Check sheet for the modelled part. Datum: model origin and axes. Units: mm. A direction names the side the tool comes from. Round coordinates to 2 decimals unless told otherwise and drop trailing zeros. Loops run counter-clockwise (first coordinate to the right, second up) from the corner with the lowest first, then second, coordinate; pieces in that order, holes last. Notation, with made-up numbers: (52.5, 72) - (81.5, 72) arc R6 ccw to (81.5, 81) - close; hole circle Ø4 at (-6, 0). An arc over 180 degrees is marked (long way). Return JSON: item names as keys, results as strings.
Autodesk Inventor part; units mm, degrees
ref_plane "YZ Plane" through (0, 0, 0) normal (1, 0, 0) x (0, 1, 0)
ref_plane "XZ Plane" through (0, 0, 0) normal (0, 1, 0) x (-1, 0, 0)
ref_plane "XY Plane" through (0, 0, 0) normal (0, 0, 1) x (1, 0, 0)
sketch "草图1" plane through (0, 0, 0) normal (0, 1, 0) x (-1, 0, 0)
  line L0 (-24, 18) -> (24, 18)
  line L1 (24, 0) -> (39.8795, 0) construction
  line L2 (-24, -18) -> (24, -18)
  arc A0 (-24, 18) -> (-24, -18) centre (0, 0) ccw
  arc A1 (24, -18) -> (24, 18) centre (0, 0) ccw
  dimension "d9" = 18
  dimension "d10" = 30
extrude "拉伸1" add sketch "草图1" along normal blind 8
sketch "草图2" plane through (0, 8, 0) normal (0, 1, 0) x (1, 0, 0)
  arc A0 (-24, 18) -> (-24, -18) centre (0, 0) ccw
  circle A1 centre (0, 0) radius 15
  dimension "d13" = 30
extrude "拉伸2" add sketch "草图2" along normal blind 27
hole "孔1" at (0, 35, 0) direction (0, -1, 0) diameter 20 end through all
ref_plane "工作平面1" through (-24, 0, 26) normal (0, 0, 1) x (1, 0, 0)
sketch "草图3" plane through (-24, 0, 26) normal (0, 0, 1) x (1, 0, 0)
  line L0 (0, 8) -> (48, 8)
  line L1 (16.5, 8) -> (16.5, 15)
  arc A0 (31.5, 15) -> (16.5, 15) centre (24, 15) ccw
  line L2 (31.5, 15) -> (31.5, 8)
  point P0 (24, 0)
  dimension "d27" = 7
  dimension "d29" = 7.5
extrude "拉伸3" add sketch "草图3" against normal up to surface
hole "孔2" at (0, 15, 26) direction (0, 0, -1) diameter 10 end up to surface
sketch "草图4" plane through (0, 0, 0) normal (1, 0, 0) x (0, 1, 0)
  line L0 (35, 10) -> (35, -10)
  line L1 (30, 5) -> (35, 5)
  line L2 (35, 5) -> (35, -5)
  line L3 (35, -5) -> (30, -5)
  line L4 (30, -5) -> (30, 5)
  line L5 (6.6641, 0) -> (11.8794, 0) construction
  point P0 (0, 0)
  dimension "d41" = 5
  dimension "d43" = 10
extrude "拉伸4" cut sketch "草图4" along normal through all both and the other way through all
properties part number "第一次上机-模型3（改）"
Q1. Tool access check on faces 1 (the face through (7.5, 12, 20)), 2 (the face through (-3.252, 21.311, -14.643)), 3 (the face through (-11, 33, -5)), 4 (the face through (0.16, 22.5, 19.59)). Record the directions out of +Z, -Z, +X, -X, +Y, -Y that give a thin tool (end or side, any length) a straight path to the whole face; none if there is none.
Answer key:
{"face 1": "+Z, +X, +Y", "face 2": "+Y", "face 3": "+X, -X, +Y", "face 4": "+Z, +Y"}
Q2. Draft check along Z on faces 5 (the face through (0, 4, 18)), 6 (the face through (12, 30, 0)), 7 (the face through (0, 8, 22)), 8 (the face through (11, 32, 5)). Enter one of: released by +Z, released by -Z, zero draft, split by the parting line, or undercut.
Answer key:
{"face 5": "released by +Z", "face 6": "undercut", "face 7": "zero draft", "face 8": "undercut"}
Q3. Sectioned sample at D-D (y = 4). Enter the section's corners in (x, z).
Answer key:
{"outline": "(-24, -18) - (24, -18) arc R30 ccw to (24, 18) - (-24, 18) arc R30 ccw to start; hole circle Ø20 at (0, 0)"}
Q4. Sectioned sample at C-C (z = 0). Enter the section's corners in (x, y).
Answer key:
{"outline": "(-30, 0) - (-10, 0) - (-10, 30) - (-15, 30) - (-15, 8) - (-30, 8) - close; (10, 0) - (30, 0) - (30, 8) - (15, 8) - (15, 30) - (10, 30) - close"}
Q5. Scan lines: probe 1 along Z at (x, y) = (0, 25.5); probe 2 along Y at (x, z) = (0, 13); probe 3 along X at (y, z) = (15, 19.25). Record each from-to range of solid material in increasing order. Write a range as [from, to].
Answer key:
{"probe 1": "z = [-15, -10], [10, 15]", "probe 2": "y = [0, 10], [20, 35]", "probe 3": "x = [-7.5, -5], [5, 7.5]"}
Q6. Sectioned sample at B-B (x = 0). Enter the section's corners in (y, z).
Answer key:
{"outline": "(0, -18) - (8, -18) - (8, -15) - (35, -15) - (35, -10) - (0, -10) - close; (0, 10) - (10, 10) - (10, 26) - (8, 26) - (8, 18) - (0, 18) - close; (20, 10) - (35, 10) - (35, 15) - (22.5, 15) - (22.5, 26) - (20, 26) - close"}
Q7. Depth check by flat-ended pin: P1, Ø12, axis at x = 0, z = 0, coming from the +Y side; P2, Ø2.5, axis at x = -12, y = 32, coming from the +Z side; P3, Ø4, axis at x = -10, y = 33.5, coming from the -Z side; P4, Ø2, axis at y = 4, z = 3, coming from the +X side. Enter the tip coordinate at first touch or a pass-through.
Answer key:
{"P1": "passes through", "P2": "stops at z = 10.46", "P3": "stops at z = -12.69", "P4": "stops at x = 29.93"}
Q8. Sectioned sample at A-A (y = 32.5). Enter the section's corners in (x, z), plus the area to 3 significant figures.
Answer key:
{"outline": "(-14.14, -5) arc R15 ccw to (14.14, -5) - (8.66, -5) arc R10 cw to (-8.66, -5) - close; (-14.14, 5) - (-8.66, 5) arc R10 cw to (8.66, 5) - (14.14, 5) arc R15 ccw to start", "area": "290 mm²"}
